Can you work these out from the model? Positions are in its coordinate system, mm. A direction names the side the tool comes from. Round coordinates to 2 decimals unless told otherwise and drop trailing zeros. Write each loop counter-clockwise with the first axis right and the second up, starting at its lowest first coordinate (ties: lowest second). Pieces come first, ordered by that corner, then holes. Notation, with made-up numbers: (68, 80) -> (89, 80) arc R23 ccw to (89, 111) -> close; hole circle Ø3 at (8.25, 13). An arc over 180 degrees is marked (long way). Use CSV: the item, a comma, the result in double quotes.
```python
from build123d import *

# Parameters (mm, degrees)
SKETCH_1_W          = 140
SKETCH_1_H          = 20
SKETCH_1_W_2        = 20
SKETCH_1_H_2        = 100
EXTRUDE_1_DEPTH     = 65
SKETCH_5_R          = 32.5
EXTRUDE_3_DEPTH     = 60
SKETCH_6_R          = 17.5
CUT_EXTRUDE_1_DEPTH = 176.87282337
SKETCH_7_R          = 15
CUT_EXTRUDE_2_DEPTH = 164.343962239
RIB_1_REACH         = 173.555
SKETCH_8_WALL_W     = 439.450580606
SKETCH_8_WALL_H     = 20


with BuildPart() as part:
    # Эскиз1 → Бобышка-Вытянуть1 (new, symmetric)
    with BuildSketch(Plane.XY):
        Rectangle(SKETCH_1_W, SKETCH_1_H)
        with Locations((60, 60)):
            Rectangle(SKETCH_1_W_2, SKETCH_1_H_2)
    extrude(amount=EXTRUDE_1_DEPTH, both=True)

    # Эскиз5 → Бобышка-Вытянуть3 (add)
    with BuildSketch(Plane(origin=(70, 0, 0), x_dir=(0, 0, -1), z_dir=(1, 0, 0))):
        with Locations((0, 110)):
            Circle(SKETCH_5_R)
    extrude(amount=-EXTRUDE_3_DEPTH)

    # Эскиз6 → Вырез-Вытянуть1 (cut, through all)
    with BuildSketch(Plane.ZY.offset(-10)):
        with Locations((0, 110)):
            Circle(SKETCH_6_R)
    extrude(amount=-CUT_EXTRUDE_1_DEPTH, mode=Mode.SUBTRACT)

    # Эскиз7 → Вырез-Вытянуть2 (cut, through all)
    with BuildSketch(Plane(origin=(0, 10, 0), x_dir=(1, 0, 0), z_dir=(0, 1, 0))):
        with Locations((-70, 0)):
            Circle(SKETCH_7_R)
    extrude(amount=-CUT_EXTRUDE_2_DEPTH, mode=Mode.SUBTRACT)

    # Эскиз8 wall → Ребро1 (add, up to next)
    with BuildSketch(Plane(origin=(10, 35, 0), x_dir=(0.847998304005, 0.529998940003, 0), z_dir=(-0.529998940003, 0.847998304005, 0)), mode=Mode.PRIVATE) as rib_1_sk1:
        Rectangle(SKETCH_8_WALL_W, SKETCH_8_WALL_H)
    rib_1_tool1 = extrude(rib_1_sk1.sketch, amount=-RIB_1_REACH, mode=Mode.PRIVATE) - part.part
    add(rib_1_tool1.solids().sort_by_distance((10, 35, 0))[0])


solid = part.part
```
Q1. On a 3-axis mill with a long thin cutter (end or side, diameter ignored), from which of +Z, -Z, +X, -X, +Y, -Y can I reach the whole of each face in a straight line? I mean faces 1 (the face through (50, 59, 15)), 2 (the face through (27, 26, -10)), 3 (the face through (60, 110, -49)). Say none if no direction works.
Resolved:
face 1,"-X"
face 2,"-Z, -X"
face 3,"-Z, +X, -X, +Y"
Q2. Suppose I cut it at A-A (z = 0). Write out the boundary of the cut face in (x, y), and give its area (3 significant figures).
Resolved:
outline,"(-55, -10) -> (70, -10) -> (70, 92.5) -> (10, 92.5) -> (10, 77.5) -> (50, 77.5) -> (50, 60) -> (-30, 10) -> (-55, 10) -> close; (10, 127.5) -> (70, 127.5) -> (70, 142.5) -> (10, 142.5) -> close"
area,"7,650 mm^2"
Q3. Will these pins go through, and if not, where does the flat tip stop? P1, Ø16, axis at x = 63, z = -56.5, coming from the +Y side; P2, Ø15, axis at x = 24, y = 45, coming from the +Z side; P3, Ø2, axis at x = -11, z = -16, coming from the +Y side.
Resolved:
P1,"stops at y = 110"
P2,"stops at z = 10"
P3,"stops at y = 10"
Q4. If we mould it in two halves opening along Z, with no side actions, what happens to faces 4 (the face through (-55, 0, 0)), 5 (the face through (-70, 0, -40)), 6 (the face through (33.753, 142.223, 4.231))? For each: released by +Z, released by -Z, zero draft, split by the parting line, or undercut.
Resolved:
face 4,"undercut"
face 5,"zero draft"
face 6,"split by the parting line"
Q5. Suppose I cut it at D-D (z = -40.5). Write out the boundary of the cut face in (x, y).
Resolved:
outline,"(-70, -10) -> (70, -10) -> (70, 110) -> (50, 110) -> (50, 10) -> (-70, 10) -> close"
Q6. Suppose I cut it at B-B (y = 38). Write out the boundary of the cut face in (x, z).
Resolved:
outline,"(14.8, -10) -> (50, -10) -> (50, -65) -> (70, -65) -> (70, 65) -> (50, 65) -> (50, 10) -> (14.8, 10) -> close"
Q7. Please list where these lines run through material, in increasing order: probe 1 along Y at (x, z) = (40, 0); probe 2 along Y at (x, z) = (27, 15); probe 3 along X at (y, z) = (107.5, -40).
Resolved:
probe 1,"y = -10 to 53.75, 77.5 to 92.5, 127.5 to 142.5"
probe 2,"y = -10 to 10, 81.17 to 100.99, 119.01 to 138.83"
probe 3,"x = 50 to 70"
Q8. Suppose I cut it at C-C (y = 121.5). Write out the boundary of the cut face in (x, z).
Resolved:
outline,"(10, -30.4) -> (70, -30.4) -> (70, -13.19) -> (10, -13.19) -> close; (10, 13.19) -> (70, 13.19) -> (70, 30.4) -> (10, 30.4) -> close"
